Model file for the job. Use its own axes, mm. A direction names the side the tool comes from. Give positions to 0.01 mm unless a question says otherwise; leave off trailing zeros. Write each loop counter-clockwise with the first axis right and the second up, starting at its lowest first coordinate (ties: lowest second). Pieces come first, ordered by that corner, then holes.
```python
from build123d import *

# Parameters (mm, degrees)
SKETCH1_R               = 24
BOSS_EXTRUDE1_DEPTH     = 4
SKETCH2_W               = 10
SKETCH2_H               = 10
BOSS_EXTRUDE2_DEPTH     = 8
SKETCH4_R               = 1.4
CUT_EXTRUDE2_DEPTH      = 4
CUT_EXTRUDE3_DEPTH      = 35.871191548
CUT_EXTRUDE3_DEPTH_BACK = 35.871191548


with BuildPart() as part:
    # Sketch1 → Boss-Extrude1 (new body)
    with BuildSketch(Plane(origin=(0, 0, 0), x_dir=(1, 0, 0), z_dir=(0, 1, 0))):
        with Locations(Location((0, 0, 0), (0, 0, 270))):
            Circle(SKETCH1_R)
        with BuildLine():
            Line((2, 1.5), (2, -1.5))
            ThreePointArc((2, -1.5), (-2.5, 0), (2, 1.5))
        make_face(mode=Mode.SUBTRACT)
    extrude(amount=BOSS_EXTRUDE1_DEPTH)

    # Sketch2 → Boss-Extrude2 (add)
    with BuildSketch(Plane(origin=(0, 4, 0), x_dir=(1, 0, 0), z_dir=(0, 1, 0))):
        Rectangle(SKETCH2_W, SKETCH2_H)
    extrude(amount=BOSS_EXTRUDE2_DEPTH)

    # Sketch4 → Cut-Extrude2 (cut)
    with BuildSketch(Plane(origin=(5, 0, 0), x_dir=(0, 0, -1), z_dir=(1, 0, 0))):
        with Locations((0, 8)):
            Circle(SKETCH4_R)
    extrude(amount=-CUT_EXTRUDE2_DEPTH, mode=Mode.SUBTRACT)

    # Sketch3 → Cut-Extrude3 (cut, two sides: drawn at the far end of the back side and taken through both)
    with BuildSketch(Plane.XZ.offset(-4).offset(-CUT_EXTRUDE3_DEPTH_BACK)):
        with BuildLine():
            Line((2, -1.661324773), (2, 1.661324773))
            ThreePointArc((2, 1.661324773), (-2.6, 0), (2, -1.661324773))
        make_face()
    extrude(amount=CUT_EXTRUDE3_DEPTH + CUT_EXTRUDE3_DEPTH_BACK, mode=Mode.SUBTRACT)


solid = part.part
```
1. Slice it at B-B, the plane y = 5.25. Write the cut outline in (x, z), and give its area (3 significant figures).
Calculated:
outline: (-5, -5) - (5, -5) - (5, 5) - (-5, 5) - close; hole (2, -1.66) - (2, 1.66) arc R2.6 ccw (long way) to start
area: 80.1 mm2
2. Pin check, flat tips, straight feed: P1, Ø10, axis at x = -11.5, z = 16.5, coming from the -Y side; P2, Ø2, axis at x = -12.5, z = -10.5, coming from the +Y side; P3, Ø2.5, axis at x = 1, y = 10, coming from the +Z side; P4, Ø4, axis at y = 9, z = 1, coming from the +X side. Stop position of each tip, or through.
Calculated:
P1: stops at y = 0
P2: stops at y = 4
P3: stops at z = 5
P4: stops at x = 5
3. Pull direction Y, two halves, no side cores. Call faces 4 (the cylindrical face through (7.21, 1.97, 22.89)), 5 (the flat face through (2.2, 12, -0.1)), 6 (the cylindrical face through (3.521, 6.633, 0.303)), 7 (the flat face through (0, 0, 5)): +Y half, -Y half, draft (parallel to the pull), parting line (faces both ways), or undercut.
Calculated:
face 4: draft
face 5: +Y half
face 6: undercut
face 7: -Y half
4. Which spindle directions (+Z, -Z, +X, -X, +Y, -Y) get a long thin tool onto all of the face, cutting with end or side? Do faces 1 (the flat face through (0, 8, 5)), 2 (the flat face through (5, 6, 0)), 3 (the flat face through (-5, 8, 0)). Say none if no direction does.
Calculated:
face 1: +Z, +X, -X, +Y
face 2: +Z, -Z, +X, +Y
face 3: +Z, -Z, -X, +Y
5. Slice it at A-A, the plane x = 0. Write the cut outline in (y, z).
Calculated:
outline: (0, -24) - (4, -24) - (4, -5) - (12, -5) - (12, -2.6) - (0, -2.6) - close; (0, 2.6) - (12, 2.6) - (12, 5) - (4, 5) - (4, 24) - (0, 24) - close
6. Probe probe 1 along X at (y, z) = (3.75, 0); probe 2 along Y at (x, z) = (3.75, 0); probe 3 along Z at (x, y) = (0, 7). List the from-to ranges inside material, lowest first.
Calculated:
probe 1: x = -24 to -2.6, 2 to 24
probe 2: y = 0 to 6.6, 9.4 to 12
probe 3: z = -5 to -2.6, 2.6 to 5
7. Slice it at D-D, the plane z = 20.5. Write the cut outline in (x, y).
Calculated:
outline: (-12.48, 0) - (12.48, 0) - (12.48, 4) - (-12.48, 4) - close
8. Slice it at C-C, the plane y = 8. Write the cut outline in (x, z), and give its area (3 significant figures).
Calculated:
outline: (-5, -5) - (5, -5) - (5, -1.4) - (2, -1.4) - (2, -1.66) arc R2.6 cw (long way) to (2, 1.66) - (2, 1.4) - (5, 1.4) - (5, 5) - (-5, 5) - close
area: 71.7 mm2
